from build123d import *

# Parameters (mm, degrees)
F0_R     = 12.5
F1_DEPTH = 2
F2_R     = 1.7334803781
F3_DEPTH = 25


with BuildPart() as f1:
    # F0 (on Top) → F1 (new body)
    with BuildSketch(Plane.XY):
        with BuildLine():
            Line((14.9999987334, -9.0138802964), (14.9999987334, 9.0138802964))
            ThreePointArc((14.9999987334, 9.0138802964), (-17.5, 0), (14.9999987334, -9.0138802964))
        make_face()
        Circle(F0_R, mode=Mode.SUBTRACT)
        with BuildLine():
            ThreePointArc((14.9999987334, -9.0138802964), (16.8634216254, -4.6770729183), (17.5, 0))
            ThreePointArc((17.5, 0), (16.8634216254, 4.6770729183), (14.9999987334, 9.0138802964))
            Line((14.9999987334, 9.0138802964), (14.9999987334, -9.0138802964))
        make_face()
        with BuildLine():
            ThreePointArc((14.9999987334, 9.0138802964), (16.8634216254, 4.6770729183), (17.5, 0))
            ThreePointArc((17.5, 0), (16.8634216254, -4.6770729183), (14.9999987334, -9.0138802964))
            Line((14.9999987334, -9.0138802964), (14.9999987334, -17.5000000745))
            Line((14.9999987334, -17.5000000745), (19.9999987334, -17.5000000745))
            Line((19.9999987334, -17.5000000745), (19.9999987334, 17.4999999255))
            Line((19.9999987334, 17.4999999255), (14.9999987334, 17.4999999255))
            Line((14.9999987334, 17.4999999255), (14.9999987334, 9.0138802964))
        make_face()
    extrude(amount=F1_DEPTH)

    # F2 (on face) → F3 (join)
    with BuildSketch(Plane.XY.offset(2)):
        with Locations((16.8318804353, 15.2465272695)):
            Circle(F2_R)
    extrude(amount=F3_DEPTH)


solid = f1.part
Input: part model. Units: mm. Frame: model coordinates. A direction names the side the tool comes from. Give positions to 0.01 mm unless a question says otherwise; leave off trailing zeros. Loops run counter-clockwise (first coordinate to the right, second up) from the corner with the lowest first, then second, coordinate; pieces in that order, holes last. Notation, with made-up numbers: M 16.25,-10 L 45.25,-10 A37 cw 45.25,26 Z; hole C 48.5,0.5 d11. An arc over 180 degrees is marked long. Use one line per item in the form item = value.
1. First-contact query: pin 1 (0.6 mm diameter, centred on y = 12.5, z = 1, fed in from -X); pin 2 (4 mm diameter, centred on x = 12, y = -11.5, fed in from +Z); pin 3 (8 mm diameter, centred on x = -10, z = 4.5, fed in from +Y). Flat tips, straight axial feed; report the tip coordinate or a pass-through.
Numbers:
pin_1 = -12.55
pin_2 = 2
pin_3 = 16.09
2. Section query A-A, the plane x = 0. Return the cut outline in (y, z).
Numbers:
outline = M -17.5,0 L -12.5,0 L -12.5,2 L -17.5,2 Z; M 12.5,0 L 17.5,0 L 17.5,2 L 12.5,2 Z
3. Section query B-B, the plane y = -4. Return the cut outline in (x, z), and give its area (3 significant figures).
Numbers:
outline = M -17.04,0 L -11.84,0 L -11.84,2 L -17.04,2 Z; M 11.84,0 L 20,0 L 20,2 L 11.84,2 Z
area = 26.7 mm²
4. Line query: L1, parallel to Y at x = 0, z = 1.55; L2, parallel to Z at x = 8, y = -11.5; L3, parallel to X at y = 16, z = 2.75. Output: solid intervals per line, ascending.
Numbers:
L1 = -17.5 to -12.5, 12.5 to 17.5
L2 = 0 to 2
L3 = 15.27 to 18.39
5. Reachability of faces 4 (the face through (15, 13, 1)), 5 (the face through (18, 17.5, 1)) from +Z, -Z, +X, -X, +Y, -Y: full face, straight path, thin tool, end or side. Return the list, or none.
Numbers:
face_4 = +Z, -Z, +Y
face_5 = +Z, -Z, +X, -X, +Y
6. Section query D-D, the plane z = 24.5. Return the cut outline in (x, y).
Numbers:
outline = C 16.83,15.25 d3.47
7. Section query C-C, the plane y = 14.5. Return the cut outline in (x, z).
Numbers:
outline = M -9.8,0 L 9.8,0 L 9.8,2 L -9.8,2 Z; M 15,0 L 20,0 L 20,2 L 18.4,2 L 18.4,27 L 15.27,27 L 15.27,2 L 15,2 Z
8. Pull-direction query (X, two-part tool) for faces 1 (the face through (18.485, 15.767, 14.325)), 2 (the face through (20, 0, 1)), 3 (the face through (15, -13, 1)); classes: released by +X, released by -X, zero draft, split by the parting line, or undercut.
Numbers:
face_1 = split by the parting line
face_2 = released by +X
face_3 = undercut
